```python
from build123d import *

# Parameters (mm, degrees)
SKETCH_1_R          = 4
SKETCH_1_R_2        = 1.383428465
SKETCH_1_R_3        = 1.5
SKETCH_1_R_4        = 2
EXTRUDE_1_DEPTH     = 2
SKETCH_2_W          = 8
SKETCH_2_H          = 2
SKETCH_2_W_2        = 42
EXTRUDE_2_DEPTH     = 25
FILLET_1_R          = 2
SKETCH_3_R          = 4
SKETCH_3_R_2        = 1.5
CUT_EXTRUDE_2_DEPTH = 2
FILLET_2_R          = 2
SKETCH_4_R          = 2
CUT_EXTRUDE_3_DEPTH = 90


with BuildPart() as part:
    # 草图1 → 凸台-拉伸1 (new body)
    with BuildSketch(Plane(origin=(0, 0, 0), x_dir=(1, 0, 0), z_dir=(0, 1, 0))):
        with BuildLine():
            Line((-17, 17.25), (17, 17.25))
            ThreePointArc((17, 17.25), (18.414213562, 16.664213562), (19, 15.25))
            Line((19, 15.25), (19, 7.25))
            Line((19, 7.25), (21, 7.25))
            Line((21, 7.25), (21, 12.25))
            Line((21, 12.25), (29, 12.25))
            Line((29, 12.25), (29, -10.25))
            ThreePointArc((29, -10.25), (28.121320344, -12.371320344), (26, -13.25))
            Line((26, -13.25), (21, -13.25))
            Line((21, -13.25), (21, -20.25))
            Line((21, -20.25), (-21, -20.25))
            Line((-21, -20.25), (-21, -13.25))
            Line((-21, -13.25), (-26, -13.25))
            ThreePointArc((-26, -13.25), (-28.121320344, -12.371320344), (-29, -10.25))
            Line((-29, -10.25), (-29, 12.25))
            Line((-29, 12.25), (-21, 12.25))
            Line((-21, 12.25), (-21, 7.25))
            Line((-21, 7.25), (-19, 7.25))
            Line((-19, 7.25), (-19, 15.25))
            ThreePointArc((-19, 15.25), (-18.414213562, 16.664213562), (-17, 17.25))
        make_face()
        with Locations(Location((0, -8.25, 0), (0, 0, 270))):
            Circle(SKETCH_1_R, mode=Mode.SUBTRACT)
        with Locations(Location((0, -1.25, 0), (0, 0, 270))):
            Circle(SKETCH_1_R_2, mode=Mode.SUBTRACT)
        with Locations(Location((-7, -8.25, 0), (0, 0, 270))):
            Circle(SKETCH_1_R_3, mode=Mode.SUBTRACT)
        with Locations(Location((0, -15.25, 0), (0, 0, 270))):
            Circle(SKETCH_1_R_3, mode=Mode.SUBTRACT)
        with Locations(Location((7, -8.25, 0), (0, 0, 270))):
            Circle(SKETCH_1_R_3, mode=Mode.SUBTRACT)
        with Locations(Location((-10.5, 2.25, 0), (0, 0, 270))):
            Circle(SKETCH_1_R, mode=Mode.SUBTRACT)
        with Locations(Location((-10.5, 9.25, 0), (0, 0, 270))):
            Circle(SKETCH_1_R_3, mode=Mode.SUBTRACT)
        with Locations(Location((-3.5, 2.25, 0), (0, 0, 270))):
            Circle(SKETCH_1_R_3, mode=Mode.SUBTRACT)
        with Locations(Location((-17.5, 2.25, 0), (0, 0, 270))):
            Circle(SKETCH_1_R_3, mode=Mode.SUBTRACT)
        with Locations(Location((-10.5, -4.75, 0), (0, 0, 270))):
            Circle(SKETCH_1_R_3, mode=Mode.SUBTRACT)
        with Locations(Location((10.5, -4.75, 0), (0, 0, 90))):
            Circle(SKETCH_1_R_3, mode=Mode.SUBTRACT)
        with Locations(Location((3.5, 2.25, 0), (0, 0, 90))):
            Circle(SKETCH_1_R_3, mode=Mode.SUBTRACT)
        with Locations(Location((17.5, 2.25, 0), (0, 0, 90))):
            Circle(SKETCH_1_R_3, mode=Mode.SUBTRACT)
        with Locations(Location((10.5, 9.25, 0), (0, 0, 90))):
            Circle(SKETCH_1_R_3, mode=Mode.SUBTRACT)
        with Locations(Location((10.5, 2.25, 0), (0, 0, 90))):
            Circle(SKETCH_1_R, mode=Mode.SUBTRACT)
        with Locations(Location((-24, 2.25, 0), (0, 0, 270))):
            Circle(SKETCH_1_R_4, mode=Mode.SUBTRACT)
        with Locations(Location((24, 2.25, 0), (0, 0, 270))):
            Circle(SKETCH_1_R_4, mode=Mode.SUBTRACT)
        with Locations(Location((-24, -7.75, 0), (0, 0, 270))):
            Circle(SKETCH_1_R_4, mode=Mode.SUBTRACT)
        with Locations(Location((24, -7.75, 0), (0, 0, 270))):
            Circle(SKETCH_1_R_4, mode=Mode.SUBTRACT)
    extrude(amount=EXTRUDE_1_DEPTH)

    # 草图2 → 凸台-拉伸2 (add)
    with BuildSketch(Plane(origin=(0, 2, 0), x_dir=(1, 0, 0), z_dir=(0, 1, 0))):
        with Locations((-25, 11.25)):
            Rectangle(SKETCH_2_W, SKETCH_2_H)
        with Locations((0, -19.25)):
            Rectangle(SKETCH_2_W_2, SKETCH_2_H)
        with Locations((25, 11.25)):
            Rectangle(SKETCH_2_W, SKETCH_2_H)
    extrude(amount=EXTRUDE_2_DEPTH)

    # 圆角1
    fillet_1_edges = [part.edges().sort_by_distance(p)[0] for p in [
        (0, 0, 20.25),
        (-25, 0, -12.25),
        (25, 0, -12.25),
    ]]
    fillet(fillet_1_edges, radius=FILLET_1_R)

    # 草图3 → 切除-拉伸2 (cut)
    with BuildSketch(Plane.XY.offset(20.25)):
        with Locations((-10.5, 14.5)):
            Circle(SKETCH_3_R)
        with Locations((-10.5, 21.5)):
            Circle(SKETCH_3_R_2)
        with Locations((-17.5, 14.5)):
            Circle(SKETCH_3_R_2)
        with Locations((-3.5, 14.5)):
            Circle(SKETCH_3_R_2)
        with Locations((-10.5, 7.5)):
            Circle(SKETCH_3_R_2)
        with Locations(Location((17.5, 14.5, 0), (0, 0, 180))):
            Circle(SKETCH_3_R_2)
        with Locations(Location((10.5, 14.5, 0), (0, 0, 180))):
            Circle(SKETCH_3_R)
        with Locations(Location((3.5, 14.5, 0), (0, 0, 180))):
            Circle(SKETCH_3_R_2)
        with Locations(Location((10.5, 21.5, 0), (0, 0, 180))):
            Circle(SKETCH_3_R_2)
        with Locations(Location((10.5, 7.5, 0), (0, 0, 180))):
            Circle(SKETCH_3_R_2)
        with BuildLine():
            Line((-19, 27), (19, 27))
            ThreePointArc((19, 27), (20.414213562, 26.414213562), (21, 25))
            Line((21, 25), (21, 28.113497729))
            Line((21, 28.113497729), (-21, 28.113497729))
            Line((-21, 28.113497729), (-21, 25))
            ThreePointArc((-21, 25), (-20.414213562, 26.414213562), (-19, 27))
        make_face()
    extrude(amount=-CUT_EXTRUDE_2_DEPTH, mode=Mode.SUBTRACT)

    # 圆角2
    fillet_2_edges = [part.edges().sort_by_distance(p)[0] for p in [
        (-29, 27, -11.25),
        (-21, 27, -11.25),
        (29, 27, -11.25),
        (21, 27, -11.25),
    ]]
    fillet(fillet_2_edges, radius=FILLET_2_R)

    # 草图4 → 切除-拉伸3 (cut)
    with BuildSketch(Plane(origin=(0, 0, -12.25), x_dir=(-1, 0, 0), z_dir=(0, 0, -1))):
        with Locations((-25, 20)):
            Circle(SKETCH_4_R)
        with Locations((-25, 10)):
            Circle(SKETCH_4_R)
        with Locations((25, 20)):
            Circle(SKETCH_4_R)
        with Locations((25, 10)):
            Circle(SKETCH_4_R)
    extrude(amount=-CUT_EXTRUDE_3_DEPTH, mode=Mode.SUBTRACT)


solid = part.part
```
Input: part model. Units: mm. Frame: model coordinates. Coordinates: 2 decimals unless noted, no trailing zeros. Write each loop counter-clockwise with the first axis right and the second up, starting at its lowest first coordinate (ties: lowest second). Pieces come first, ordered by that corner, then holes.
1) Section B-B on z = -9.25. Output: boundary loops of the cut face in (x, y).
2) Material intervals for line 1 along X through (y, z) = (0.65, -9.25); line 2 along Y through (x, z) = (25, -11); line 3 along Z through (x, y) = (22, 24), sorted ascending.
3) Mould query, pull axis Z, two halves, no side actions, for faces 1 (the flat face through (25, 27, -11)), 2 (the cylindrical face through (22.783, 0.986, 6.163)), 3 (the cylindrical face through (18.4, 0.99, -16.68)), 4 (the flat face through (0, 14, 20.25)). Classes: pulls with the +Z half, pulls with the -Z half, needs draft (parallel to the pull), parting line crosses it, or undercut.
4) Section C-C on x = -13. Output: boundary loops of the cut face in (y, z), and give its area (3 significant figures).
5) Pin query (flat end, axial travel): pin 1 Ø3.5 at (x, y) = (-10.5, 21.5) entering from -Z; pin 2 Ø6 at (x, z) = (-5.5, -4) entering from +Y; pin 3 Ø2 at (x, y) = (23, 1) entering from +Z. Return the tip coordinate at first contact, or that it passes through.
6) Section D-D on x = 24. Output: boundary loops of the cut face in (y, z), and give its area (3 significant figures).
7) Section A-A on y = 3.75. Output: boundary loops of the cut face in (x, z).
Check result:
1. outline: (-29, 0) - (-21, 0) - (-21, 2) - (-29, 2) - close; (-19, 0) - (-12, 0) - (-12, 2) - (-19, 2) - close; (-9, 0) - (9, 0) - (9, 2) - (-9, 2) - close; (12, 0) - (19, 0) - (19, 2) - (12, 2) - close; (21, 0) - (29, 0) - (29, 2) - (21, 2) - close
2. line 1: x = -29 to -21, -19 to -12, -9 to 9, 12 to 19, 21 to 29
2. line 2: y = 0.15 to 8, 12 to 18, 22 to 27
2. line 3: z = -12.25 to -10.25
3. face 1: needs draft
3. face 2: undercut
3. face 3: pulls with the -Z half
3. face 4: pulls with the +Z half
4. outline: (0, -17.25) - (2, -17.25) - (2, -5.37) - (0, -5.37) - close; (0, 0.87) - (2, 0.87) - (2, 18.25) - (11.38, 18.25) - (11.38, 20.25) - (2, 20.25) arc R2 ccw to (0, 18.25) - close; (17.62, 18.25) - (27, 18.25) - (27, 20.25) - (17.62, 20.25) - close
4. area: 99.2 mm2
5. pin 1: stops at z = 18.25
5. pin 2: stops at y = 2
5. pin 3: stops at z = 13.25
6. outline: (0, -10.25) arc R2 ccw to (2, -12.25) - (8.27, -12.25) - (8.27, -10.25) - (2, -10.25) - (2, -4.25) - (0, -4.25) - close; (0, -0.25) - (2, -0.25) - (2, 5.75) - (0, 5.75) - close; (0, 9.75) - (2, 9.75) - (2, 13.25) - (0, 13.25) - close; (11.73, -12.25) - (18.27, -12.25) - (18.27, -10.25) - (11.73, -10.25) - close; (21.73, -12.25) - (27, -12.25) - (27, -10.25) - (21.73, -10.25) - close
6. area: 70.3 mm2
7. outline: (-29, -12.25) - (-21, -12.25) - (-21, -10.25) - (-29, -10.25) - close; (-21, 18.25) - (21, 18.25) - (21, 20.25) - (-21, 20.25) - close; (21, -12.25) - (29, -12.25) - (29, -10.25) - (21, -10.25) - close
